Answer from the drawing. Dimensions are ordinates in mm from the lowest x, y and z of the part. A direction names the side the tool comes from. Coordinates: 2 decimals unless noted, no trailing zeros. Order: outer loops, then holes, each group sorted by start corner. A loop starts at its lowest first (then second) coordinate and runs counter-clockwise, first axis right, second up. Notation, with made-up numbers: (-32, 60.5) - (-1, 60.5) arc R15 ccw to (-1, 68.5) - close; hole circle Ø6 at (-7.5, 76.25). An arc over 180 degrees is marked (long way). Use a Markdown table: item, result. Add a question column.
Item 1: Find the intervals of material crossed by line 1 along Y through (x, z) = (46, 44); line 2 along Z through (x, y) = (40.5, 69); line 3 along X through (y, z) = (74, 78), in increasing order.
Item 2: The part is cut by section C-C, the plane z = 79. Give the vertices of the cut face in (x, y).
Item 3: For the marked faces 1, 2 and 3, determine the directions among +Z, -Z, +X, -X, +Y, -Y from which every point of the face is accessible in a straight line to the end or side of a thin tool.
Item 4: The mould has two halves that part along Z. Classify the marked faces 4, 5, 6 and 7: released by +Z, released by -Z, zero draft, split by the parting line, or undercut.
Item 5: The part is cut by section D-D, the plane y = 89. Give the vertices of the cut face in (x, z).
Item 6: Flat-ended cylindrical pins translate along their axes: P1, Ø13, axis at x = 42.5, z = 77, coming from the +Y side; P2, Ø6, axis at y = 73, z = 12, coming from the -X side; P3, Ø5, axis at x = 51, z = 68, coming from the +Y side; P4, Ø3, axis at y = 40, z = 15.5, coming from the -X side. Find the tip coordinate at first contact, or state that the pin passes through.
Item 7: The part is cut by section A-A, the plane x = 33. Give the vertices of the cut face in (y, z).
Item 8: The part is cut by section B-B, the plane y = 71.5. Give the vertices of the cut face in (x, z).
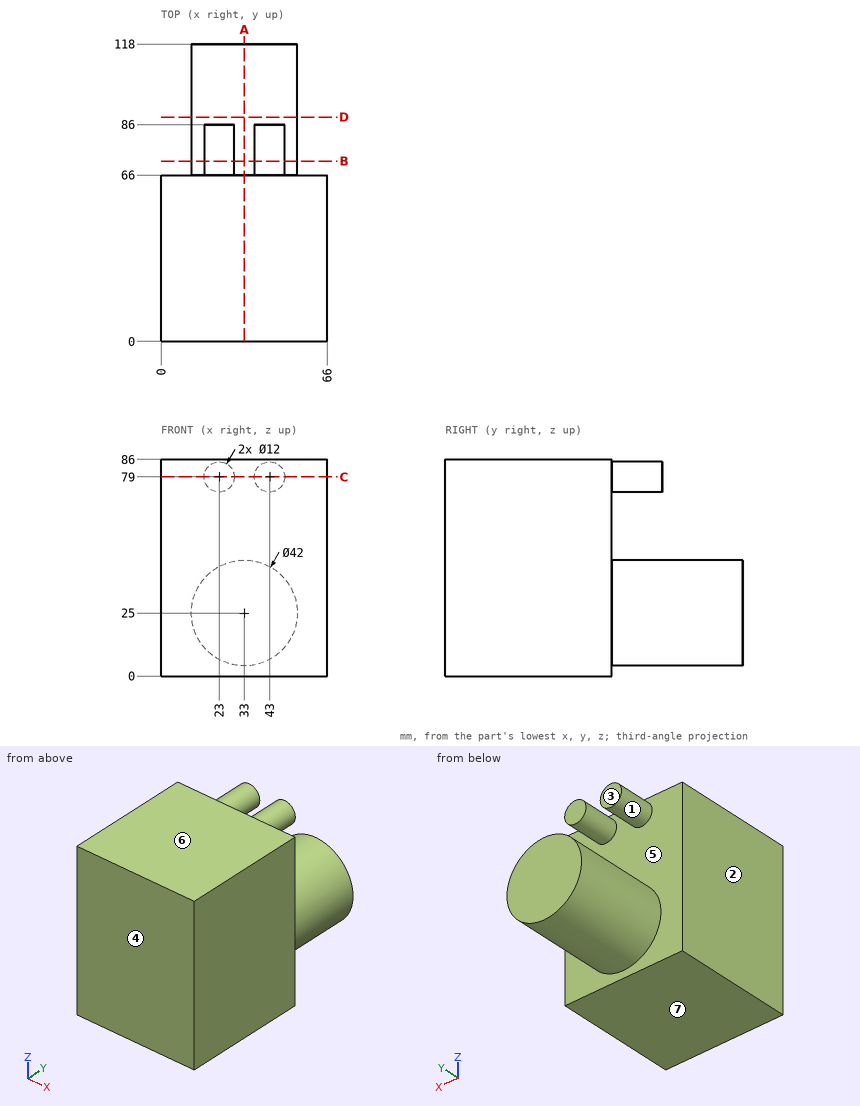
Solution:
| question | item | result |
|---|---|---|
| 1 | line 1 | y = 0 to 66 |
| 1 | line 2 | z = 5.38 to 44.62, 73.55 to 84.45 |
| 1 | line 3 | x = 17.08 to 28.92, 37.08 to 48.92 |
| 2 | outline | (0, 0) - (66, 0) - (66, 66) - (49, 66) - (49, 86) - (37, 86) - (37, 66) - (29, 66) - (29, 86) - (17, 86) - (17, 66) - (0, 66) - close |
| 3 | face 1 | +Y |
| 3 | face 2 | +Z, -Z, -X, +Y, -Y |
| 3 | face 3 | +Z, +X, -X, +Y |
| 4 | face 4 | zero draft |
| 4 | face 5 | undercut |
| 4 | face 6 | released by +Z |
| 4 | face 7 | released by -Z |
| 5 | outline | circle Ø42 at (33, 25) |
| 6 | P1 | stops at y = 86 |
| 6 | P2 | stops at x = 14.53 |
| 6 | P3 | stops at y = 66 |
| 6 | P4 | stops at x = 0 |
| 7 | outline | (0, 0) - (66, 0) - (66, 4) - (118, 4) - (118, 46) - (66, 46) - (66, 86) - (0, 86) - close |
| 8 | outline | circle Ø42 at (33, 25); circle Ø12 at (23, 79); circle Ø12 at (43, 79) |
